```python
from build123d import *

# Parameters (mm, degrees)
SKETCH1_W           = 100
SKETCH1_H           = 60
SKETCH1_R           = 6.5
BOSS_EXTRUDE1_DEPTH = 4
SKETCH2_R           = 4.5
CUT_EXTRUDE1_DEPTH  = 5


with BuildPart() as part:
    # Sketch1 → Boss-Extrude1 (new body)
    with BuildSketch(Plane(origin=(0, 0, 0), x_dir=(1, 0, 0), z_dir=(0, 1, 0))):
        Rectangle(SKETCH1_W, SKETCH1_H)
        Circle(SKETCH1_R, mode=Mode.SUBTRACT)
    extrude(amount=BOSS_EXTRUDE1_DEPTH)

    # Sketch2 → Cut-Extrude1 (cut, through all)
    with BuildSketch(Plane(origin=(0, 4, 0), x_dir=(1, 0, 0), z_dir=(0, 1, 0))):
        with Locations((-41, 21)):
            Circle(SKETCH2_R)
        with Locations((41, 21)):
            Circle(SKETCH2_R)
        with Locations((41, -21)):
            Circle(SKETCH2_R)
        with Locations((-41, -21)):
            Circle(SKETCH2_R)
    extrude(amount=-CUT_EXTRUDE1_DEPTH, mode=Mode.SUBTRACT)


solid = part.part
```
Here's how the part is built. I have some questions about the finished solid (model axes, mm). Give positions to 0.01 mm unless a question says otherwise; leave off trailing zeros. Write each loop counter-clockwise with the first axis right and the second up, starting at its lowest first coordinate (ties: lowest second). Pieces come first, ordered by that corner, then holes.
(1) Imagine slicing it at C-C, the plane y = 1.75. Write out the boundary of the cut face in (x, z).
Output values:
outline: (-50, -30) - (50, -30) - (50, 30) - (-50, 30) - close; hole circle Ø9 at (-41, -21); hole circle Ø9 at (-41, 21); hole circle Ø13 at (0, 0); hole circle Ø9 at (41, -21); hole circle Ø9 at (41, 21)
(2) If I drill on L1, parallel to Z at x = -41, y = 1.9; L2, parallel to X at y = 1.8, z = 21; L3, parallel to X at y = 1.35, z = 0, over which ranges is the centre line in solid material (lowest first)?
Output values:
L1: z = -30 to -25.5, -16.5 to 16.5, 25.5 to 30
L2: x = -50 to -45.5, -36.5 to 36.5, 45.5 to 50
L3: x = -50 to -6.5, 6.5 to 50
(3) Imagine slicing it at A-A, the plane x = 41. Write out the boundary of the cut face in (y, z), and give its area (3 significant figures).
Output values:
outline: (0, -30) - (4, -30) - (4, -25.5) - (0, -25.5) - close; (0, -16.5) - (4, -16.5) - (4, 16.5) - (0, 16.5) - close; (0, 25.5) - (4, 25.5) - (4, 30) - (0, 30) - close
area: 168 mm2
(4) Thinking about a two-plate mould opening in Z: for faces 1 (the face through (-1, 2, 30)), 2 (the face through (-1, 2, -30)), 3 (the face through (-5.158, 1.972, 3.955)), 4 (the face through (-38.581, 2.028, 17.206)), which applies, pulls with the +Z half, pulls with the -Z half, needs draft (parallel to the pull), parting line crosses it, or undercut?
Output values:
face 1: pulls with the +Z half
face 2: pulls with the -Z half
face 3: undercut
face 4: undercut
(5) Imagine slicing it at B-B, the plane z = 21. Write out the boundary of the cut face in (x, y), and give its area (3 significant figures).
Output values:
outline: (-50, 0) - (-45.5, 0) - (-45.5, 4) - (-50, 4) - close; (-36.5, 0) - (36.5, 0) - (36.5, 4) - (-36.5, 4) - close; (45.5, 0) - (50, 0) - (50, 4) - (45.5, 4) - close
area: 328 mm2
